Check sheet for the modelled part. Datum: model origin and axes. Units: mm. Face numbers are marked on the shaded views. A direction names the side the tool comes from. Give positions to 0.01 mm unless a question says otherwise; leave off trailing zeros. Write each loop counter-clockwise with the first axis right and the second up, starting at its lowest first coordinate (ties: lowest second). Pieces come first, ordered by that corner, then holes. Notation, with made-up numbers: M 12,17.25 L 41,17.25 A8 ccw 41,24.25 Z; hole C -23,-38.5 d10. An arc over 180 degrees is marked long. Write item = value, one per line. Start each with the question number.
1) Cross-section at B-B, the plane y = -2. Record the cut outline in (x, z).
2) Cross-section at A-A, the plane z = 15. Record the cut outline in (x, y).
3) Cross-section at D-D, the plane x = 0. Record the cut outline in (y, z), plus the area to 3 significant figures.
4) Cross-section at C-C, the plane x = 6. Record the cut outline in (y, z), plus the area to 3 significant figures.
5) Scan lines: line 1 along X through (y, z) = (-0.25, -8); line 2 along X through (y, z) = (-5.75, 10.5); line 3 along Y through (x, z) = (-7.25, -10). Record each from-to range of solid material in increasing order. Write a range as [from, to].
6) Access from +Z, -Z, +X, -X, +Y, -Y to the whole of each face (thin tool, end or side, straight path). Record for the marked faces 1 and 2.
7) Go/stop test with flat-tipped pins: pin 1 (6.5 mm diameter, centred on x = -2, y = 2.5, fed in from -Z); pin 2 (1.5 mm diameter, centred on y = -5.5, z = 15, fed in from +X); pin 3 (3 mm diameter, centred on x = -5.5, z = 18.5, fed in from +Y). Record where each tip stops, or that it passes through.
```python
from build123d import *

# Parameters (mm, degrees)
F0_R      = 9.5
F1_DEPTH  = 20
F3_DEPTH  = 50
F5_DEPTH  = 50
F7_DEPTH  = 2.5
F8_R      = 11
F8_R_2    = 9.5
F9_DEPTH  = 39
F10_R     = 11
F10_R_2   = 9.5
F11_DEPTH = 16


with BuildPart() as f1:
    # F0 (on Top) → F1 (new body, symmetric)
    with BuildSketch(Plane.XY):
        Circle(F0_R)
    extrude(amount=F1_DEPTH, both=True)

    # F2 (on face) → F3 (cut)
    with BuildSketch(Plane.XY.offset(20)):
        with BuildLine():
            Line((-1.0508030978, 1.2395313024), (-1.0508030978, 7.9306880439))
            ThreePointArc((-1.0508030978, 7.9306880439), (-5.5890325577, 5.7238723841), (-7.9033892825, 1.2395313024))
            Line((-7.9033892825, 1.2395313024), (-1.0508030978, 1.2395313024))
        make_face()
        with BuildLine():
            Line((1.0508030978, 1.2395313024), (7.9033892825, 1.2395313024))
            ThreePointArc((7.9033892825, 1.2395313024), (5.5890325577, 5.7238723841), (1.0508030978, 7.9306880439))
            Line((1.0508030978, 7.9306880439), (1.0508030978, 1.2395313024))
        make_face()
        with BuildLine():
            ThreePointArc((1.0508030978, -7.9306880439), (5.5890325577, -5.7238723841), (7.9033892825, -1.2395313024))
            Line((7.9033892825, -1.2395313024), (1.0508030978, -1.2395313024))
            Line((1.0508030978, -1.2395313024), (1.0508030978, -7.9306880439))
        make_face()
        with BuildLine():
            ThreePointArc((-7.9033892825, -1.2395313024), (-5.5890325577, -5.7238723841), (-1.0508030978, -7.9306880439))
            Line((-1.0508030978, -7.9306880439), (-1.0508030978, -1.2395313024))
            Line((-1.0508030978, -1.2395313024), (-7.9033892825, -1.2395313024))
        make_face()
    extrude(amount=-F3_DEPTH, mode=Mode.SUBTRACT)

    # F4 (on face) + F2 (on face) → F5 (cut)
    with BuildSketch(Plane.XY.offset(20)):
        with BuildLine():
            Line((-7.9033892825, 1.2395313024), (-1.0508030978, 1.2395313024))
            Line((-1.0508030978, 1.2395313024), (-1.0508030978, 7.9306880439))
            ThreePointArc((-1.0508030978, 7.9306880439), (-5.5890325577, 5.7238723841), (-7.9033892825, 1.2395313024))
        make_face()
        with BuildLine():
            ThreePointArc((-1.0508030978, -1.2395313024), (-1.625, 0), (-1.0508030978, 1.2395313024))
            Line((-1.0508030978, 1.2395313024), (-7.9033892825, 1.2395313024))
            ThreePointArc((-7.9033892825, 1.2395313024), (-8, 0), (-7.9033892825, -1.2395313024))
            Line((-7.9033892825, -1.2395313024), (-1.0508030978, -1.2395313024))
        make_face()
        with BuildLine():
            Line((-1.0508030978, 7.9306880439), (-1.0508030978, 1.2395313024))
            ThreePointArc((-1.0508030978, 1.2395313024), (0, 1.625), (1.0508030978, 1.2395313024))
            Line((1.0508030978, 1.2395313024), (1.0508030978, 7.9306880439))
            ThreePointArc((1.0508030978, 7.9306880439), (0, 8), (-1.0508030978, 7.9306880439))
        make_face()
        with BuildLine():
            Line((1.0508030978, 7.9306880439), (1.0508030978, 1.2395313024))
            Line((1.0508030978, 1.2395313024), (7.9033892825, 1.2395313024))
            ThreePointArc((7.9033892825, 1.2395313024), (5.5890325577, 5.7238723841), (1.0508030978, 7.9306880439))
        make_face()
        with BuildLine():
            Line((7.9033892825, 1.2395313024), (1.0508030978, 1.2395313024))
            ThreePointArc((1.0508030978, 1.2395313024), (1.474479575, 0.6830336617), (1.625, 0))
            ThreePointArc((1.625, 0), (1.474479575, -0.6830336617), (1.0508030978, -1.2395313024))
            Line((1.0508030978, -1.2395313024), (7.9033892825, -1.2395313024))
            ThreePointArc((7.9033892825, -1.2395313024), (7.9758107506, -0.6216452928), (8, 0))
            ThreePointArc((8, 0), (7.9758107506, 0.6216452928), (7.9033892825, 1.2395313024))
        make_face()
        with BuildLine():
            ThreePointArc((1.0508030978, -1.2395313024), (0, -1.625), (-1.0508030978, -1.2395313024))
            Line((-1.0508030978, -1.2395313024), (-1.0508030978, -7.9306880439))
            ThreePointArc((-1.0508030978, -7.9306880439), (0, -8), (1.0508030978, -7.9306880439))
            Line((1.0508030978, -7.9306880439), (1.0508030978, -1.2395313024))
        make_face()
        with BuildLine():
            Line((-1.0508030978, -7.9306880439), (-1.0508030978, -1.2395313024))
            Line((-1.0508030978, -1.2395313024), (-7.9033892825, -1.2395313024))
            ThreePointArc((-7.9033892825, -1.2395313024), (-5.5890325577, -5.7238723841), (-1.0508030978, -7.9306880439))
        make_face()
        with BuildLine():
            Line((7.9033892825, -1.2395313024), (1.0508030978, -1.2395313024))
            Line((1.0508030978, -1.2395313024), (1.0508030978, -7.9306880439))
            ThreePointArc((1.0508030978, -7.9306880439), (5.5890325577, -5.7238723841), (7.9033892825, -1.2395313024))
        make_face()
    with BuildSketch(Plane.XY.offset(20)):
        with BuildLine():
            ThreePointArc((1.625, 0), (1.474479575, 0.6830336617), (1.0508030978, 1.2395313024))
            ThreePointArc((1.0508030978, 1.2395313024), (0, 1.625), (-1.0508030978, 1.2395313024))
            ThreePointArc((-1.0508030978, 1.2395313024), (-1.625, 0), (-1.0508030978, -1.2395313024))
            ThreePointArc((-1.0508030978, -1.2395313024), (0, -1.625), (1.0508030978, -1.2395313024))
            ThreePointArc((1.0508030978, -1.2395313024), (1.474479575, -0.6830336617), (1.625, 0))
        make_face()
    extrude(amount=-F5_DEPTH, mode=Mode.SUBTRACT)

    # F6 (on face) → F7 (join)
    with BuildSketch(Plane.XY.offset(20)):
        with BuildLine():
            ThreePointArc((-1.0508030978, -1.2395313024), (-1.625, 0), (-1.0508030978, 1.2395313024))
            Line((-1.0508030978, 1.2395313024), (-7.9033892825, 1.2395313024))
            ThreePointArc((-7.9033892825, 1.2395313024), (-8, 0), (-7.9033892825, -1.2395313024))
            Line((-7.9033892825, -1.2395313024), (-1.0508030978, -1.2395313024))
        make_face()
        with BuildLine():
            Line((-1.0508030978, 7.9306880439), (-1.0508030978, 1.2395313024))
            ThreePointArc((-1.0508030978, 1.2395313024), (0, 1.625), (1.0508030978, 1.2395313024))
            Line((1.0508030978, 1.2395313024), (1.0508030978, 7.9306880439))
            ThreePointArc((1.0508030978, 7.9306880439), (0, 8), (-1.0508030978, 7.9306880439))
        make_face()
        with BuildLine():
            ThreePointArc((1.0508030978, 1.2395313024), (0, 1.625), (-1.0508030978, 1.2395313024))
            ThreePointArc((-1.0508030978, 1.2395313024), (-1.625, 0), (-1.0508030978, -1.2395313024))
            ThreePointArc((-1.0508030978, -1.2395313024), (0, -1.625), (1.0508030978, -1.2395313024))
            ThreePointArc((1.0508030978, -1.2395313024), (1.474479575, -0.6830336617), (1.625, 0))
            ThreePointArc((1.625, 0), (1.474479575, 0.6830336617), (1.0508030978, 1.2395313024))
        make_face()
        with BuildLine():
            Line((7.9033892825, 1.2395313024), (1.0508030978, 1.2395313024))
            ThreePointArc((1.0508030978, 1.2395313024), (1.474479575, 0.6830336617), (1.625, 0))
            ThreePointArc((1.625, 0), (1.474479575, -0.6830336617), (1.0508030978, -1.2395313024))
            Line((1.0508030978, -1.2395313024), (7.9033892825, -1.2395313024))
            ThreePointArc((7.9033892825, -1.2395313024), (8, 0), (7.9033892825, 1.2395313024))
        make_face()
        with BuildLine():
            ThreePointArc((1.0508030978, -1.2395313024), (0, -1.625), (-1.0508030978, -1.2395313024))
            Line((-1.0508030978, -1.2395313024), (-1.0508030978, -7.9306880439))
            ThreePointArc((-1.0508030978, -7.9306880439), (0, -8), (1.0508030978, -7.9306880439))
            Line((1.0508030978, -7.9306880439), (1.0508030978, -1.2395313024))
        make_face()
    extrude(amount=-F7_DEPTH)

    # F8 (on face) → F9 (join)
    with BuildSketch(Plane(origin=(0, 0, -20), x_dir=(1, 0, 0), z_dir=(0, 0, -1))):
        Circle(F8_R)
        Circle(F8_R_2, mode=Mode.SUBTRACT)
    extrude(amount=-F9_DEPTH)

    # F10 (on face) → F11 (cut)
    with BuildSketch(Plane(origin=(0, 0, -20), x_dir=(1, 0, 0), z_dir=(0, 0, -1))):
        Circle(F10_R)
        Circle(F10_R_2, mode=Mode.SUBTRACT)
    extrude(amount=-F11_DEPTH, mode=Mode.SUBTRACT)


solid = f1.part
```
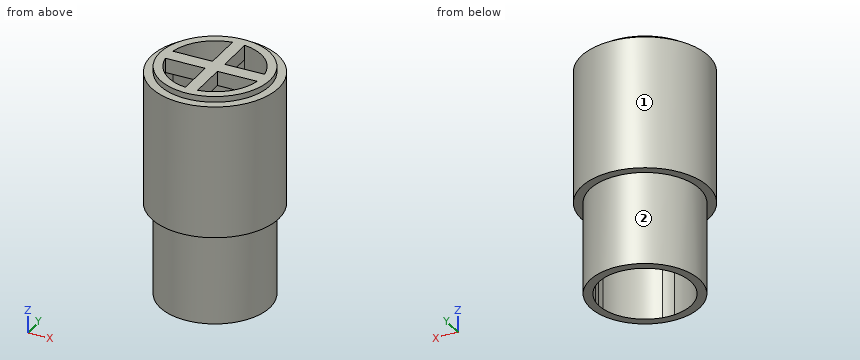
Reply:
q1.outline = M -10.82,-4 L -9.29,-4 L -9.29,-20 L -7.75,-20 L -7.75,20 L -9.29,20 L -9.29,19 L -10.82,19 Z; M -1.05,17.5 L 1.05,17.5 L 1.05,20 L -1.05,20 Z; M 7.75,-20 L 9.29,-20 L 9.29,-4 L 10.82,-4 L 10.82,19 L 9.29,19 L 9.29,20 L 7.75,20 Z
q2.outline = C 0,0 d22; hole C 0,0 d16
q3.outline = M -11,-4 L -9.5,-4 L -9.5,-20 L -8,-20 L -8,17.5 L 8,17.5 L 8,-20 L 9.5,-20 L 9.5,-4 L 11,-4 L 11,19 L 9.5,19 L 9.5,20 L -9.5,20 L -9.5,19 L -11,19 Z
q3.area = 229 mm2
q4.outline = M -9.22,-4 L -7.37,-4 L -7.37,-20 L -5.29,-20 L -5.29,20 L -7.37,20 L -7.37,19 L -9.22,19 Z; M -1.24,17.5 L 1.24,17.5 L 1.24,20 L -1.24,20 Z; M 5.29,-20 L 7.37,-20 L 7.37,-4 L 9.22,-4 L 9.22,19 L 7.37,19 L 7.37,20 L 5.29,20 Z
q4.area = 257 mm2
q5.line_1 = [-9.5, -8], [8, 9.5]
q5.line_2 = [-9.38, -5.56], [5.56, 9.38]
q5.line_3 = [-6.14, -3.38], [3.38, 6.14]
q6.face_1 = +Z, -Z
q6.face_2 = -Z
q7.pin_1 = 17.5
q7.pin_2 = 9.92
q7.pin_3 = 10.25
